from build123d import *

# Parameters (mm, degrees)
F0_R     = 12.5
F1_DEPTH = 20
F3_DEPTH = 5
F4_DEPTH = 4
F5_R     = 8
F6_R     = 3


with BuildPart() as f1:
    # F0 (on Top) → F1 (new body)
    with BuildSketch(Plane.XY):
        Circle(F0_R)
        with BuildLine():
            ThreePointArc((-9.1651513899, -4), (-10, 0), (-9.1651513899, 4))
            Line((-9.1651513899, 4), (-4.472135955, 4))
            ThreePointArc((-4.472135955, 4), (-4.2426406871, 4.2426406871), (-4, 4.472135955))
            Line((-4, 4.472135955), (-4, 9.1651513899))
            ThreePointArc((-4, 9.1651513899), (0, 10), (4, 9.1651513899))
            Line((4, 9.1651513899), (4, 4.472135955))
            ThreePointArc((4, 4.472135955), (4.2426406871, 4.2426406871), (4.472135955, 4))
            Line((4.472135955, 4), (9.1651513899, 4))
            ThreePointArc((9.1651513899, 4), (10, 0), (9.1651513899, -4))
            Line((9.1651513899, -4), (4.472135955, -4))
            ThreePointArc((4.472135955, -4), (4.2426406871, -4.2426406871), (4, -4.472135955))
            Line((4, -4.472135955), (4, -9.1651513899))
            ThreePointArc((4, -9.1651513899), (0, -10), (-4, -9.1651513899))
            Line((-4, -9.1651513899), (-4, -4.472135955))
            ThreePointArc((-4, -4.472135955), (-4.2426406871, -4.2426406871), (-4.472135955, -4))
            Line((-4.472135955, -4), (-9.1651513899, -4))
        make_face(mode=Mode.SUBTRACT)
    extrude(amount=F1_DEPTH)

    # F2 (on Top) → F3 (join)
    with BuildSketch(Plane.XY):
        with BuildLine():
            ThreePointArc((10, -7.5), (11.8585412256, -3.9528470752), (12.5, 0))
            ThreePointArc((12.5, 0), (11.8585412256, 3.9528470752), (10, 7.5))
            ThreePointArc((10, 7.5), (-12.5, 0), (10, -7.5))
        make_face()
        with BuildLine():
            ThreePointArc((10, 7.5), (11.8585412256, 3.9528470752), (12.5, 0))
            ThreePointArc((12.5, 0), (11.8585412256, -3.9528470752), (10, -7.5))
            Line((10, -7.5), (89.9234008285, -4))
            Line((89.9234008285, -4), (89.9234008285, 0))
            Line((89.9234008285, 0), (89.9234008285, 4))
            Line((89.9234008285, 4), (10, 7.5))
        make_face()
    extrude(amount=-F3_DEPTH)

    # F2 (on Top) → F4 (join)
    with BuildSketch(Plane.XY):
        with BuildLine():
            ThreePointArc((10, -7.5), (11.8585412256, -3.9528470752), (12.5, 0))
            ThreePointArc((12.5, 0), (11.8585412256, 3.9528470752), (10, 7.5))
            ThreePointArc((10, 7.5), (-12.5, 0), (10, -7.5))
        make_face()
        with BuildLine():
            ThreePointArc((10, 7.5), (11.8585412256, 3.9528470752), (12.5, 0))
            ThreePointArc((12.5, 0), (11.8585412256, -3.9528470752), (10, -7.5))
            Line((10, -7.5), (89.9234008285, -4))
            Line((89.9234008285, -4), (89.9234008285, 0))
            Line((89.9234008285, 0), (89.9234008285, 4))
            Line((89.9234008285, 4), (10, 7.5))
        make_face()
    extrude(amount=-F4_DEPTH)

    # F5
    f5_edges = [f1.edges().sort_by_distance(p)[0] for p in [
        (10, 7.5, -2.5),
        (10, -7.5, -2.5),
    ]]
    fillet(f5_edges, radius=F5_R)

    # F6
    f6_edges = [f1.edges().sort_by_distance(p)[0] for p in [
        (89.923401, 4, -2.5),
        (89.923401, -4, -2.5),
    ]]
    fillet(f6_edges, radius=F6_R)


solid = f1.part
Part model, mm, in its own coordinate system. A direction names the side the tool comes from. Round coordinates to 2 decimals unless told otherwise and drop trailing zeros. Write each loop counter-clockwise with the first axis right and the second up, starting at its lowest first coordinate (ties: lowest second). Pieces come first, ordered by that corner, then holes. Notation, with made-up numbers: M 19.25,41.5 L 50.25,41.5 A34 cw 50.25,71.5 Z; hole C 88,22 d4. An arc over 180 degrees is marked long. Return JSON: item names as keys, results as strings. Group by question number.
(1) Which spindle directions (+Z, -Z, +X, -X, +Y, -Y) get a long thin tool onto all of the face, cutting with end or side? Do faces 4 (the face through (4, 7, 10)), 5 (the face through (5, -5, 20)). Say none if no direction does.
(2) Saw through at D-D on y = 0. Write the cut outline in (x, z).
(3) Two-plate mould, pull along Y, no slides. Class faces 1 (the face through (49.629, -5.765, -2.465)), 2 (the face through (0, -10, 10)), 3 (the face through (49, 0, 0)): +Y half, -Y half, draft (parallel to the pull), parting line (faces both ways), or undercut.
(4) Saw through at A-A on z = 3.25. Write the cut outline in (x, y), then the cut area to 3 significant figures.
(5) Saw through at B-B on x = 0. Write the cut outline in (y, z).
(6) Pin check, flat tips, straight feed: pin 1 Ø5 at (y, z) = (-4.5, -1) entering from +X; pin 2 Ø1.4 at (y, z) = (-6.5, 9) entering from +X; pin 3 Ø2.5 at (y, z) = (7.5, 10) entering from +X. Stop position of each tip, or through.
(7) Drill centre lines: probe 1 along Y at (x, z) = (8.5, 16.75); probe 2 along X at (y, z) = (-0.25, 12); probe 3 along Z at (x, y) = (3, -6.25). Where is each one in solid material? Low to high.
(8) Saw through at C-C on z = -1. Write the cut outline in (x, y).
Returned:
{
 "1": {"face 4": "+Z", "face 5": "+Z, +X, -X, +Y, -Y"},
 "2": {"outline": "M -12.5,-5 L 89.92,-5 L 89.92,0 L 12.5,0 L 12.5,20 L 10,20 L 10,0 L -10,0 L -10,20 L -12.5,20 Z"},
 "3": {"face 1": "-Y half", "face 2": "undercut", "face 3": "draft"},
 "4": {"outline": "C 0,0 d25; hole M -9.17,-4 L -4.47,-4 A6 ccw -4,-4.47 L -4,-9.17 A10 ccw 4,-9.17 L 4,-4.47 A6 ccw 4.47,-4 L 9.17,-4 A10 ccw 9.17,4 L 4.47,4 A6 ccw 4,4.47 L 4,9.17 A10 ccw -4,9.17 L -4,4.47 A6 ccw -4.47,4 L -9.17,4 A10 ccw Z", "area": "243 mm²"},
 "5": {"outline": "M -12.5,-5 L 12.5,-5 L 12.5,20 L 10,20 L 10,0 L -10,0 L -10,20 L -12.5,20 Z"},
 "6": {"pin 1": "x = 89.79", "pin 2": "x = 11.07", "pin 3": "x = 10.83"},
 "7": {"probe 1": "-9.17 to -4, 4 to 9.17", "probe 2": "-12.5 to -10, 10 to 12.5", "probe 3": "-5 to 0"},
 "8": {"outline": "M 8.28,-9.36 A8 cw 13.24,-7.36 L 87.05,-4.13 A3 ccw 89.92,-1.13 L 89.92,1.13 A3 ccw 87.05,4.13 L 13.24,7.36 A8 cw 8.28,9.36 A12.5 ccw long Z"}
}
